Autodesk Inventor part; units mm, degrees
ref_plane "YZ Plane" through (0, 0, 0) normal (1, 0, 0) x (0, 1, 0)
ref_plane "XZ Plane" through (0, 0, 0) normal (0, 1, 0) x (-1, 0, 0)
ref_plane "XY Plane" through (0, 0, 0) normal (0, 0, 1) x (1, 0, 0)
sketch "Sketch1" plane through (0, 0, 0) normal (0, 0, 1) x (1, 0, 0)
  line L0 (280, 76) -> (280, 66) construction
  line L1 (280, 76) -> (274, 76) construction
  line L2 (274, 76) -> (274, 66) construction
  line L3 (280, 66) -> (274, 66) construction
  line L4 (280, 16) -> (280, 6) construction
  line L5 (280, 16) -> (274, 16) construction
  line L6 (274, 16) -> (274, 6) construction
  line L7 (280, 6) -> (274, 6) construction
  line L8 (235, 6) -> (235, 0) construction
  line L9 (235, 0) -> (280, 0) construction
  line L10 (280, 0) -> (280, 6) construction
  line L11 (235, 6) -> (280, 6) construction
  line L12 (95, 6) -> (95, 0) construction
  line L13 (95, 0) -> (185, 0) construction
  line L14 (185, 0) -> (185, 6) construction
  line L15 (95, 6) -> (185, 6) construction
  line L16 (45, 0) -> (45, 6) construction
  line L17 (0, 6) -> (45, 6) construction
  line L18 (0, 0) -> (0, 6) construction
  line L19 (0, 0) -> (45, 0) construction
  line L20 (0, 16) -> (0, 6) construction
  line L21 (0, 6) -> (6, 6) construction
  line L22 (6, 16) -> (6, 6) construction
  line L23 (0, 16) -> (6, 16) construction
  line L24 (0, 76) -> (0, 66) construction
  line L25 (0, 66) -> (6, 66) construction
  line L26 (6, 76) -> (6, 66) construction
  line L27 (0, 76) -> (6, 76) construction
  line L28 (274, 16) -> (280, 16)
  line L29 (280, 16) -> (280, 66)
  line L30 (280, 66) -> (274, 66)
  line L31 (6, 16) -> (0, 16)
  line L32 (0, 16) -> (0, 66)
  line L33 (0, 66) -> (6, 66)
  line L34 (95, 6) -> (95, 0)
  line L35 (95, 0) -> (45, 0)
  line L36 (45, 0) -> (45, 6)
  line L37 (185, 6) -> (185, 0)
  line L38 (185, 0) -> (235, 0)
  line L39 (235, 0) -> (235, 6)
  line L40 (274, 76) -> (274, 66)
  line L41 (274, 16) -> (274, 6)
  line L42 (274, 6) -> (235, 6)
  line L43 (185, 6) -> (95, 6)
  line L44 (45, 6) -> (6, 6)
  line L45 (6, 6) -> (6, 16)
  line L46 (6, 66) -> (6, 76)
  line L47 (45, 76) -> (45, 61)
  line L48 (45, 61) -> (235, 61)
  line L49 (235, 61) -> (235, 76)
  line L50 (6, 76) -> (45, 76)
  line L51 (235, 76) -> (274, 76)
extrude "Extrusion1" add sketch "Sketch1" against normal blind 6
chamfer "Chamfer1" distance 15 angle 45 2 edges at (45, 61, -3) (235, 61, -3)
sketch "Sketch2" plane through (0, 0, 0) normal (0, 0, 1) x (1, 0, 0)
  circle A0 centre (250, 46) radius 10
  line L0 (235, 76) -> (274, 76)
  line L1 (280, 66) -> (280, 16)
  point P0 (0, 0)
  dimension "d6" = 20
  dimension "d7" = 30
  dimension "d8" = 30
extrude "Extrusion2" cut sketch "Sketch2" against normal blind 6
properties part number "Lateral"
Design review of the part built by this model. Coordinates are the model's own, in mm. A direction names the side the tool comes from. Coordinates: 2 decimals unless noted, no trailing zeros. Loops run counter-clockwise (first coordinate to the right, second up) from the corner with the lowest first, then second, coordinate; pieces in that order, holes last. Notation, with made-up numbers: M -0.75,79 L 10.25,79 A18 ccw 10.25,91 Z; hole C 28,43.25 d9. An arc over 180 degrees is marked long. Use one line per item in the form item = value.
(1) For line 1 along Y through (x, z) = (250, -1.3); line 2 along X through (y, z) = (45, -0.7); line 3 along Y through (x, z) = (172, -1.9), list the stretches that pass through material, from the lowest coordinate up. Write a range as from..to.
Return value:
line_1 = 6..36, 56..76
line_2 = 0..240.05, 259.95..280
line_3 = 6..61
(2) Consider section A-A (y = 46). Write out the cut boundary in (x, z), and give its area (3 significant figures).
Return value:
outline = M 0,-6 L 240,-6 L 240,0 L 0,0 Z; M 260,-6 L 280,-6 L 280,0 L 260,0 Z
area = 1,560 mm2
(3) Consider section B-B (x = 250). Write out the cut boundary in (y, z).
Return value:
outline = M 6,-6 L 36,-6 L 36,0 L 6,0 Z; M 56,-6 L 76,-6 L 76,0 L 56,0 Z
(4) For faces 4 (the face through (141, 6, -3)), 5 (the face through (53, 68, -3)), 6 (the face through (6, 11, -3)), list the 3-axis set-ups (+Z, -Z, +X, -X, +Y, -Y) from which the entire face can be reached by the end or side of a thin tool; tool diameter is ignored.
Return value:
face_4 = +Z, -Z, -Y
face_5 = +Z, -Z, +Y
face_6 = +Z, -Z, -X, -Y
(5) Consider section D-D (x = 19). Write out the cut boundary in (y, z).
Return value:
outline = M 6,-6 L 76,-6 L 76,0 L 6,0 Z
(6) Clearance check with flat-ended pins moving along their axes: P1, Ø3, axis at y = 13, z = -4, coming from the +X side; P2, Ø1.8, axis at x = 119.5, z = -2.5, coming from the +Y side; P3, Ø3, axis at x = 21, z = -4, coming from the -Y side. State where each tip first meets the part, or that it passes through.
Return value:
P1 = 274
P2 = 61
P3 = 6
(7) Draft analysis for pull direction X (two halves, no side actions). For faces 1 (the face through (185, 3, -3)), 2 (the face through (3, 66, -3)), 3 (the face through (6, 71, -3)), state which applies: pulls with the +X half, pulls with the -X half, needs draft (parallel to the pull), parting line crosses it, or undercut.
Return value:
face_1 = undercut
face_2 = needs draft
face_3 = pulls with the -X half
